Check sheet for the modelled part. Datum: model origin and axes. Units: mm. A direction names the side the tool comes from. Coordinates: 2 decimals unless noted, no trailing zeros. Loops run counter-clockwise (first coordinate to the right, second up) from the corner with the lowest first, then second, coordinate; pieces in that order, holes last. Notation, with made-up numbers: (5, 13.25) - (63, 13.25) arc R16 ccw to (63, 21.25) - close; hole circle Ø11 at (78.25, 38.25). An arc over 180 degrees is marked (long way). Write each question's results on one line, items separated by ' | '. Start each with the question number.
1. Cross-section at D-D (y = -33). Record the cut outline in (x, z), and give its area (3 significant figures).
2. Cross-section at B-B (y = 25.4). Record the cut outline in (x, z), and give its area (3 significant figures).
3. Cross-section at C-C (z = 1.25). Record the cut outline in (x, y), and give its area (3 significant figures).
4. Thickness scan on line 1 (X direction, y = 4, z = 1.25); line 2 (X direction, y = -13.5, z = 0.75); line 3 (X direction, y = -0.5, z = 4.25). Record the ranges inside material, lowest first. Write a range as [from, to].
5. Draft check along Y on faces 1 (the face through (-1, -26, 0)), 2 (the face through (27.56, -39.69, 1.25)), 3 (the face through (3.81, -37, 4)). Enter one of: released by +Y, released by -Y, zero draft, split by the parting line, or undercut.
6. Gauge pin test, flat ends, axial feed: P1, Ø1, axis at x = 18.5, z = 4.5, coming from the +Y side; P2, Ø23, axis at x = 4, y = -36, coming from the +Z side; P3, Ø2, axis at y = -46.5, z = 4, coming from the -X side; P4, Ø3, axis at x = 7.5, z = 1.5, coming from the +Y side. Record the tip position at first contact, or that the pin passes through.
7. Cross-section at A-A (x = 0). Record the cut outline in (y, z), and give its area (3 significant figures).
8. Tool access check on faces 4 (the face through (-0.83, -3.72, 5.71)), 5 (the face through (-27.85, -38.59, 1.25)), 6 (the face through (-3.81, -36, 4)). Record the directions out of +Z, -Z, +X, -X, +Y, -Y that give a thin tool (end or side, any length) a straight path to the whole face; none if there is none.
```python
from build123d import *

# Parameters (mm, degrees)
F0_R     = 7.62
F1_DEPTH = 2.54
F0_R_2   = 3.81
F2_DEPTH = 5.08
F3_DEPTH = 6.35


with BuildPart() as f1:
    # F0 (on Top) → F1 (new body)
    with BuildSketch(Plane.XY):
        with BuildLine():
            ThreePointArc((38.1, 0), (0, 38.1), (-38.1, 0))
            Line((-38.1, 0), (-17.309019, -78.278743))
            ThreePointArc((-17.309019, -78.278743), (0, -91.590577), (17.309019, -78.278743))
            Line((17.309019, -78.278743), (38.1, 0))
        make_face()
        with BuildLine():
            ThreePointArc((-3.81, -6.832742), (-3.962074, 6.745697), (7.8232, 0))
            ThreePointArc((7.8232, 0), (6.745697, -3.962074), (3.81, -6.832742))
            Line((3.81, -6.832742), (3.81, -66.848693))
            ThreePointArc((3.81, -66.848693), (6.745697, -69.71936), (7.8232, -73.681435))
            ThreePointArc((7.8232, -73.681435), (-3.962074, -80.427132), (-3.81, -66.848693))
            Line((-3.81, -66.848693), (-3.81, -6.832742))
        make_face(mode=Mode.SUBTRACT)
        with Locations((-18.580349, -17.318506)):
            Circle(F0_R, mode=Mode.SUBTRACT)
        with Locations((-24.127055, 7.940101)):
            Circle(F0_R, mode=Mode.SUBTRACT)
        with Locations((18.580349, -17.318506)):
            Circle(F0_R, mode=Mode.SUBTRACT)
        with Locations((0, 25.4)):
            Circle(F0_R, mode=Mode.SUBTRACT)
        with Locations((24.127055, 7.940101)):
            Circle(F0_R, mode=Mode.SUBTRACT)
    extrude(amount=F1_DEPTH)

    # F0 (on Top) → F2 (join)
    with BuildSketch(Plane.XY):
        with BuildLine():
            ThreePointArc((3.81, -6.832742), (0, -7.8232), (-3.81, -6.832742))
            Line((-3.81, -6.832742), (-3.81, -66.848693))
            ThreePointArc((-3.81, -66.848693), (0, -65.858235), (3.81, -66.848693))
            Line((3.81, -66.848693), (3.81, -6.832742))
        make_face()
        with BuildLine():
            ThreePointArc((3.81, -66.848693), (0, -65.858235), (-3.81, -66.848693))
            ThreePointArc((-3.81, -66.848693), (-3.962074, -80.427132), (7.8232, -73.681435))
            ThreePointArc((7.8232, -73.681435), (6.745697, -69.71936), (3.81, -66.848693))
        make_face()
        with Locations((0, -73.681435)):
            Circle(F0_R_2, mode=Mode.SUBTRACT)
        with BuildLine():
            ThreePointArc((3.81, -6.832742), (6.745697, -3.962074), (7.8232, 0))
            ThreePointArc((7.8232, 0), (-3.962074, 6.745697), (-3.81, -6.832742))
            ThreePointArc((-3.81, -6.832742), (0, -7.8232), (3.81, -6.832742))
        make_face()
        Circle(F0_R_2, mode=Mode.SUBTRACT)
    extrude(amount=F2_DEPTH)

    # F0 (on Top) → F3 (join)
    with BuildSketch(Plane.XY):
        with Locations((0, -73.681435)):
            Circle(F0_R_2)
        Circle(F0_R_2)
    extrude(amount=F3_DEPTH)


solid = f1.part
```
Established:
1) outline: (-29.34, 0) - (29.34, 0) - (29.34, 2.54) - (3.81, 2.54) - (3.81, 5.08) - (-3.81, 5.08) - (-3.81, 2.54) - (-29.34, 2.54) - close | area: 168 mm^2
2) outline: (-28.4, 0) - (-7.62, 0) - (-7.62, 2.54) - (-28.4, 2.54) - close; (7.62, 0) - (28.4, 0) - (28.4, 2.54) - (7.62, 2.54) - close | area: 106 mm^2
3) outline: (-38.1, 0) - (-17.31, -78.28) arc R17.91 ccw to (17.31, -78.28) - (38.1, 0) arc R38.1 ccw to start; hole circle Ø15.24 at (-24.13, 7.94); hole circle Ø15.24 at (-18.58, -17.32); hole circle Ø15.24 at (0, 25.4); hole circle Ø15.24 at (18.58, -17.32); hole circle Ø15.24 at (24.13, 7.94) | area: 6,050 mm^2
4) line 1: [-37.89, -30.65], [-17.6, 17.6], [30.65, 37.89] | line 2: [-34.51, -25.17], [-11.99, 11.99], [25.17, 34.51] | line 3: [-7.81, 7.81]
5) face 1: zero draft | face 2: released by -Y | face 3: undercut
6) P1: through | P2: z = 5.08 | P3: x = -3.81 | P4: y = 37.62
7) outline: (-91.59, 0) - (17.78, 0) - (17.78, 2.54) - (7.82, 2.54) - (7.82, 5.08) - (3.81, 5.08) - (3.81, 6.35) - (-3.81, 6.35) - (-3.81, 5.08) - (-69.87, 5.08) - (-69.87, 6.35) - (-77.49, 6.35) - (-77.49, 5.08) - (-81.5, 5.08) - (-81.5, 2.54) - (-91.59, 2.54) - close; (33.02, 0) - (38.1, 0) - (38.1, 2.54) - (33.02, 2.54) - close | area: 537 mm^2
8) face 4: +Z | face 5: +Z, -Z, -X, -Y | face 6: +Z, -X
